```python
from build123d import *

# Parameters (mm, degrees)
F0_W      = 117.348
F0_H      = 63.5
F1_DEPTH  = 35.052
F2_W      = 117.348
F2_H      = 15.748
F3_DEPTH  = 12.7
F4_W      = 41.148
F4_H      = 15.748
F4_H_2    = 19.304
F5_DEPTH  = 18.4404
F6_W      = 15.748
F6_H      = 12.7
F7_DEPTH  = 117.349
F8_W      = 15.748
F8_H      = 12.7
F9_DEPTH  = 60.452
F10_R     = 9.525
F11_DEPTH = 35.053


with BuildPart() as f1:
    # F0 (on Front) → F1 (new body)
    with BuildSketch(Plane.XZ):
        Rectangle(F0_W, F0_H)
    extrude(amount=F1_DEPTH)

    # F2 (on face) → F3 (join)
    with BuildSketch(Plane.XY.offset(31.75)):
        with Locations((0, -7.874)):
            Rectangle(F2_W, F2_H)
    extrude(amount=F3_DEPTH)

    # F4 (on face) → F5 (cut)
    with BuildSketch(Plane.XY.offset(44.45)):
        with Locations((38.1, -7.874)):
            Rectangle(F4_W, F4_H)
        with Locations((38.1, -25.4)):
            Rectangle(F4_W, F4_H_2)
    extrude(amount=-F5_DEPTH, mode=Mode.SUBTRACT)

    # F6 (on face) → F7 (cut, through all)
    with BuildSketch(Plane.YZ.offset(58.674)):
        with Locations((-7.874, -25.4)):
            Rectangle(F6_W, F6_H)
    extrude(amount=-F7_DEPTH, mode=Mode.SUBTRACT)

    # F8 (on face) → F9 (join)
    with BuildSketch(Plane.YZ.offset(58.674)):
        with Locations((-42.926, -25.4)):
            Rectangle(F8_W, F8_H)
    extrude(amount=-F9_DEPTH)

    # F10 (on face) → F11 (cut, through all)
    with BuildSketch(Plane.XZ.offset(35.052)):
        with Locations((-26.67, -0.254)):
            Circle(F10_R)
    extrude(amount=-F11_DEPTH, mode=Mode.SUBTRACT)


solid = f1.part
```
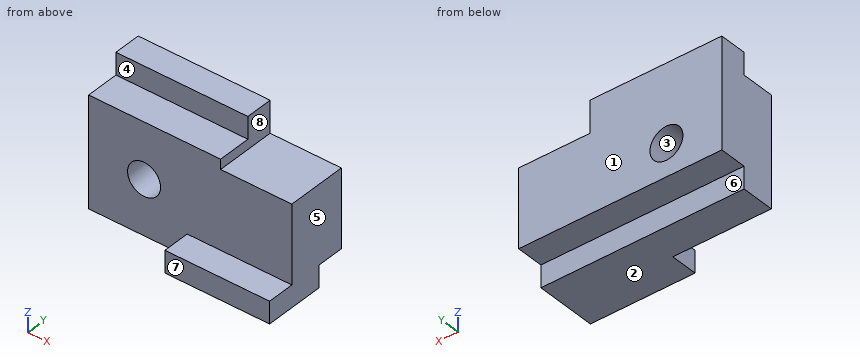
Verification items for the finished model (mm, model axes). Face numbers are marked on the shaded views. A direction names the side the tool comes from. Round coordinates to 2 decimals unless told otherwise and drop trailing zeros. Order: outer loops, then holes, each group sorted by start corner. A loop starts at its lowest first (then second) coordinate and runs counter-clockwise, first axis right, second up.
1) Cross-section at B-B, the plane z = 5. Record the cut outline in (x, y), plus the area to 3 significant figures.
Geometry says:
outline: (-58.67, -35.05) - (-34.61, -35.05) - (-34.61, 0) - (-58.67, 0) - close; (-18.73, -35.05) - (58.67, -35.05) - (58.67, 0) - (-18.73, 0) - close
area: 3,560 mm2
2) Draft check along Z on the marked faces 1, 2 and 3. Enter one of: +Z half, -Z half, draft (parallel to the pull), parting line (faces both ways), or undercut.
Geometry says:
face 1: draft
face 2: -Z half
face 3: undercut
3) Cross-section at A-A, the plane x = -26.67. Record the cut outline in (y, z).
Geometry says:
outline: (-35.05, -31.75) - (-15.75, -31.75) - (-15.75, -19.05) - (0, -19.05) - (0, -9.78) - (-35.05, -9.78) - close; (-35.05, 9.27) - (0, 9.27) - (0, 44.45) - (-15.75, 44.45) - (-15.75, 31.75) - (-35.05, 31.75) - close
4) Material ranges on line 1 (Z direction, x = -26.67, y = -12); line 2 (Z direction, x = -26, y = -12); line 3 (Y direction, x = 48, z = -13), recorded low to high.
Geometry says:
line 1: z = -19.05 to -9.78, 9.27 to 44.45
line 2: z = -19.05 to -9.76, 9.25 to 44.45
line 3: y = -35.05 to 0
5) Cross-section at C-C, the plane x = 33. Record the cut outline in (y, z).
Geometry says:
outline: (-50.8, -31.75) - (-15.75, -31.75) - (-15.75, -19.05) - (0, -19.05) - (0, 26.01) - (-35.05, 26.01) - (-35.05, -19.05) - (-50.8, -19.05) - close
6) Cross-section at D-D, the plane y = -3.5. Record the cut outline in (x, z) (3 decimals).
Geometry says:
outline: (-58.674, -19.05) - (58.674, -19.05) - (58.674, 26.01) - (17.526, 26.01) - (17.526, 44.45) - (-58.674, 44.45) - close; hole circle Ø19.05 at (-26.67, -0.254)
7) Tool access check on the marked faces 4, 5, 6, 7 and 8. Record the directions out of +Z, -Z, +X, -X, +Y, -Y that give a thin tool (end or side, any length) a straight path to the whole face; none if there is none.
Geometry says:
face 4: +Z, +X, -X, -Y
face 5: +Z, -Z, +X, +Y, -Y
face 6: -Z, +X, -X, +Y
face 7: +Z, -Z, +X, -X, -Y
face 8: +Z, +X, +Y, -Y
8) Depth check by flat-ended pin: pin 1 (4 mm diameter, centred on x = 11.5, z = -25.5, fed in from +Y); pin 2 (5 mm diameter, centred on x = -44, z = -5, fed in from -Y); pin 3 (4.5 mm diameter, centred on x = 17.5, y = -42.5, fed in from +Z). Enter the tip coordinate at first touch or a pass-through.
Geometry says:
pin 1: stops at y = -15.75
pin 2: stops at y = -35.05
pin 3: stops at z = -19.05
